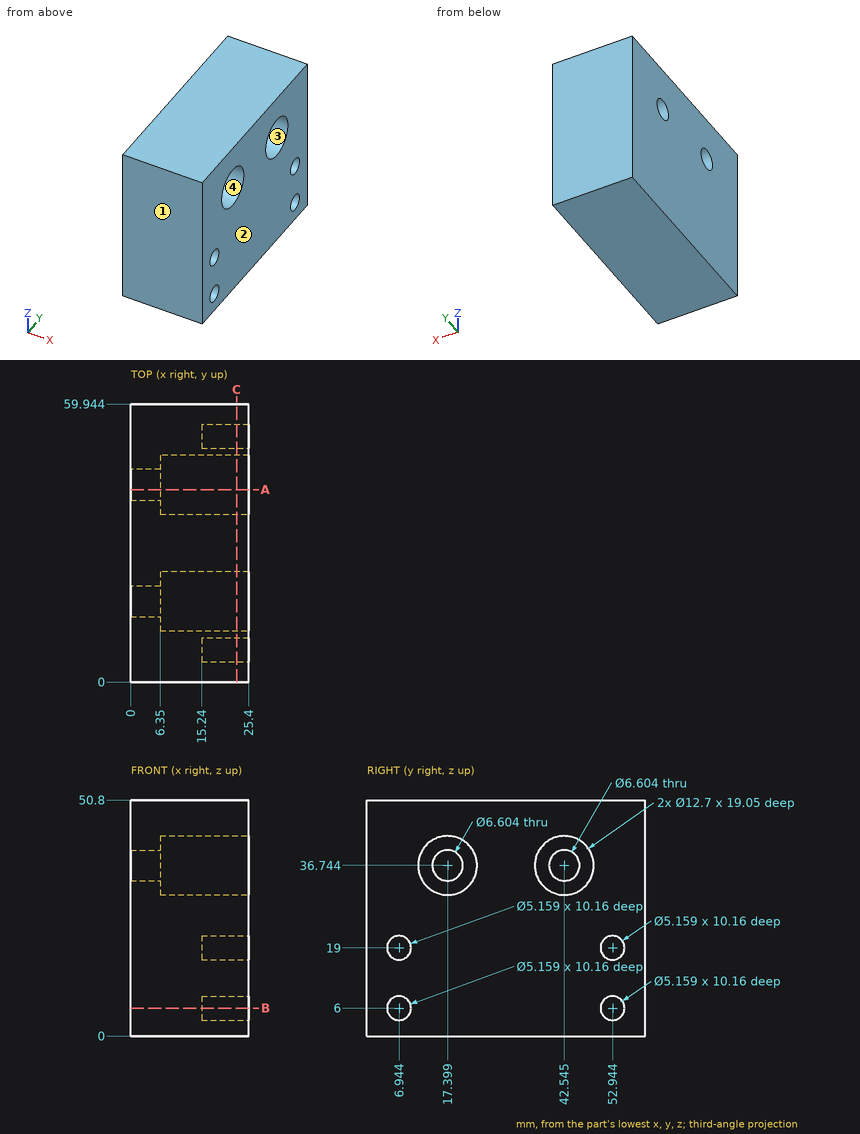
Drawing for the job (mm, zero at the part's lowest x, y, z). Coordinates: 2 decimals unless noted, no trailing zeros. Loops run counter-clockwise (first coordinate to the right, second up) from the corner with the lowest first, then second, coordinate; pieces in that order, holes last. Notation, with made-up numbers: (10.5, 51.5) - (27.5, 51.5) arc R7 cw to (27.5, 58.5) - close; hole circle Ø8 at (21, 21.5). An arc over 180 degrees is marked (long way). Use CSV: the item, a comma, the result in double quotes. Start each with the question number.
Q1. Drop flat-ended pins along their axis: P1, Ø10, axis at y = 15, z = 36.5, coming from the +X side; P2, Ø1.5, axis at y = 54, z = 19, coming from the +X side; P3, Ø8.5, axis at y = 42.54, z = 36.74, coming from the +X side. Give the stop position or say it passes through.
Q2. Probe probe 1 along Z at (x, y) = (23, 54.5); probe 2 along Y at (x, z) = (9, 33) (1 decimal); probe 3 along Z at (x, y) = (13, 45). List the from-to ranges inside material, lowest first. Write a range as from..to.
Q3. Cut at B-B, the plane z = 6. List the corners of the cut face in (x, y) (1 decimal).
Q4. Two-plate mould, pull along Y, no slides. Class the marked faces 1, 2, 3 and 4: +Y half, -Y half, draft (parallel to the pull), parting line (faces both ways), or undercut.
Q5. Cut at C-C, the plane x = 22.75. State how many separate pieces and enclosed holes the cut face has, then the cut area to 3 significant figures.
Q6. Cut at A-A, the plane y = 41.5. List the corners of the cut face in (x, z), then the cut area to 3 significant figures.
Here are the results:
1,P1,"x = 25.4"
1,P2,"x = 15.24"
1,P3,"x = 6.35"
2,probe 1,"0..3.94, 8.06..16.94, 21.06..50.8"
2,probe 2,"0..12.3, 22.5..37.4, 47.7..59.9"
2,probe 3,"0..30.89, 42.6..50.8"
3,outline,"(0, 0) - (25.4, 0) - (25.4, 4.4) - (15.2, 4.4) - (15.2, 9.5) - (25.4, 9.5) - (25.4, 50.4) - (15.2, 50.4) - (15.2, 55.5) - (25.4, 55.5) - (25.4, 59.9) - (0, 59.9) - close"
4,face 1,"-Y half"
4,face 2,"draft"
4,face 3,"undercut"
4,face 4,"undercut"
5,separate pieces,"1"
5,enclosed holes,"6"
5,area,"2,710 mm2"
6,outline,"(0, 0) - (25.4, 0) - (25.4, 30.48) - (6.35, 30.48) - (6.35, 33.61) - (0, 33.61) - close; (0, 39.88) - (6.35, 39.88) - (6.35, 43.01) - (25.4, 43.01) - (25.4, 50.8) - (0, 50.8) - close"
6,area,"1,010 mm2"
